Input: part model. Units: mm. Frame: model coordinates. Face numbers are marked on the shaded views. A direction names the side the tool comes from. Round coordinates to 2 decimals unless told otherwise and drop trailing zeros. Order: outer loops, then holes, each group sorted by start corner. A loop starts at its lowest first (then second) coordinate and runs counter-clockwise, first axis right, second up.
Item 1: Cut plane D-D on z = 9.25. Output: boundary loops of the cut face in (x, y).
Item 2: Cut plane B-B on y = 72.5. Output: boundary loops of the cut face in (x, z).
Item 3: Reachability of the marked faces 4, 5 and 6 from +Z, -Z, +X, -X, +Y, -Y: full face, straight path, thin tool, end or side. Return the list, or none.
Item 4: First-contact query: pin 1 (4 mm diameter, centred on x = -3.5, z = 12, fed in from -Y); pin 2 (2 mm diameter, centred on y = 78.5, z = 11.5, fed in from -X); pin 3 (1 mm diameter, centred on x = 5, z = 13, fed in from +Y). Flat tips, straight axial feed; report the tip coordinate or a pass-through.
Item 5: Cut plane A-A on x = -1.5. Output: boundary loops of the cut face in (y, z), then the cut area to 3 significant figures.
Item 6: Mould query, pull axis X, two halves, no side actions, for the marked faces 1, 2 and 3. Classes: released by +X, released by -X, zero draft, split by the parting line, or undercut.
Item 7: Line query: L1, parallel to Z at x = 0.5, y = 63; L2, parallel to X at y = 76, z = 14; L3, parallel to Z at x = -6, y = 67. Output: solid intervals per line, ascending.
Item 8: Cut plane C-C on x = -13. Output: boundary loops of the cut face in (y, z), then the cut area to 3 significant figures.
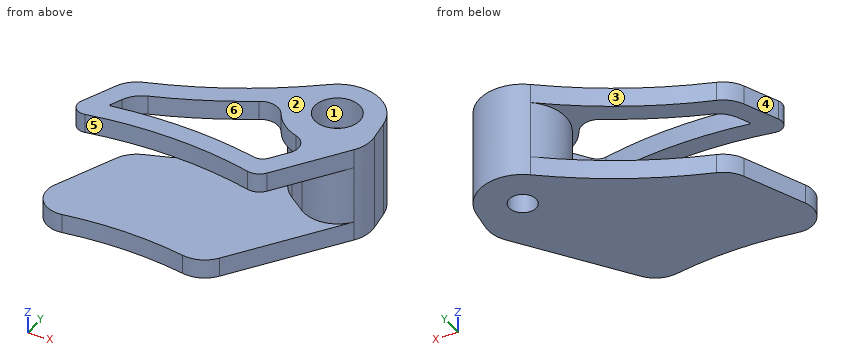
```python
from build123d import *

# Parameters (mm, degrees)
BOSS_EXTRUDE1_DEPTH     = 15
SKETCH16_R              = 2.1
CUT_EXTRUDE2_DEPTH      = 89.504764277
SKETCH17_R              = 3.5
CUT_EXTRUDE3_DEPTH      = 5
CUT_EXTRUDE1_DEPTH      = 5
CUT_EXTRUDE1_DEPTH_BACK = 4
CUT_EXTRUDE5_DEPTH      = 3
CUT_EXTRUDE4_DEPTH      = 3


with BuildPart() as part:
    # Sketch14 → Boss-Extrude1 (new body)
    with BuildSketch(Plane.XY):
        with BuildLine():
            Line((-16.161413536, 57.977264022), (-12.181084948, 67.464973009))
            ThreePointArc((-12.181084948, 67.464973009), (-11.065698538, 69.072353645), (-9.393028071, 70.087209723))
            ThreePointArc((-9.393028071, 70.087209723), (2.046505069, 75.260844547), (12.392283809, 82.373810035))
            ThreePointArc((12.392283809, 82.373810035), (19.046410902, 83.46789097), (23.273577081, 78.213798608))
            Line((23.273577081, 78.213798608), (23.760338244, 74.979563376))
            ThreePointArc((23.760338244, 74.979563376), (23.681286202, 72.988596756), (22.8727833, 71.167465139))
            Line((22.8727833, 71.167465139), (11.475608136, 54.751856173))
            ThreePointArc((11.475608136, 54.751856173), (9.468702378, 53.12015601), (6.90080904, 52.810252891))
            ThreePointArc((6.90080904, 52.810252891), (-2.49021647, 53.523672844), (-11.865953559, 52.631550555))
            ThreePointArc((-11.865953559, 52.631550555), (-15.60520233, 54.025568594), (-16.161413536, 57.977264022))
        make_face()
    extrude(amount=BOSS_EXTRUDE1_DEPTH)

    # Sketch16 → Cut-Extrude2 (cut, through all)
    with BuildSketch(Plane.XY.offset(15)):
        with Locations((16.657019892, 77.21798883)):
            Circle(SKETCH16_R)
    extrude(amount=-CUT_EXTRUDE2_DEPTH, mode=Mode.SUBTRACT)

    # Sketch17 → Cut-Extrude3 (cut)
    with BuildSketch(Plane.XY.offset(15)):
        with Locations((16.657019892, 77.21798883)):
            Circle(SKETCH17_R)
    extrude(amount=-CUT_EXTRUDE3_DEPTH, mode=Mode.SUBTRACT)

    # Sketch15 → Cut-Extrude1 (cut, two sides: drawn at the far end of the back side and taken through both)
    with BuildSketch(Plane.XY.offset(7).offset(-CUT_EXTRUDE1_DEPTH_BACK)):
        with BuildLine():
            Line((13.708420325, 83.2243377), (11.92660987, 87.484761825))
            Line((11.92660987, 87.484761825), (-22.331697338, 87.484761825))
            Line((-22.331697338, 87.484761825), (-22.331697338, 56.566228638))
            Line((-22.331697338, 56.566228638), (-22.331697338, 46.478853626))
            Line((-22.331697338, 46.478853626), (13.179214544, 46.478853626))
            Line((13.179214544, 46.478853626), (31.832474143, 71.167465139))
            Line((31.832474143, 71.167465139), (22.8727833, 71.167465139))
            ThreePointArc((22.8727833, 71.167465139), (19.43169391, 68.968964182), (15.448675977, 69.869003519))
            Line((15.448675977, 69.869003519), (12.782241645, 71.763031479))
            ThreePointArc((12.782241645, 71.763031479), (9.987686622, 77.756932137), (13.708420325, 83.2243377))
        make_face()
    extrude(amount=CUT_EXTRUDE1_DEPTH + CUT_EXTRUDE1_DEPTH_BACK, mode=Mode.SUBTRACT)

    # Sketch19 → Cut-Extrude5 (cut)
    with BuildSketch(Plane.XY.offset(15)):
        with BuildLine():
            Line((-14.431982215, 62.099622447), (-17.748305782, 61.423635141))
            Line((-17.748305782, 61.423635141), (-17.748305782, 50.845501907))
            Line((-17.748305782, 50.845501907), (18.748185883, 50.845501907))
            Line((18.748185883, 50.845501907), (18.748185883, 60.53099213))
            Line((18.748185883, 60.53099213), (15.487998108, 60.53099213))
            ThreePointArc((15.487998108, 60.53099213), (14.424069998, 59.689920639), (13.072075611, 59.582890491))
            ThreePointArc((13.072075611, 59.582890491), (0.311109574, 60.999206641), (-12.463639277, 59.713128338))
            ThreePointArc((-12.463639277, 59.713128338), (-14.168682333, 60.311811806), (-14.431982215, 62.099622447))
        make_face()
    extrude(amount=-CUT_EXTRUDE5_DEPTH, mode=Mode.SUBTRACT)

    # Sketch18 → Cut-Extrude4 (cut)
    with BuildSketch(Plane.XY.offset(15)):
        with BuildLine():
            Line((-9.882439649, 65.189392999), (-10.64394248, 63.374237016))
            ThreePointArc((-10.64394248, 63.374237016), (-10.620440593, 63.202263891), (-10.458545604, 63.139677097))
            ThreePointArc((-10.458545604, 63.139677097), (0.83913118, 63.994498661), (12.110509679, 62.84373919))
            ThreePointArc((12.110509679, 62.84373919), (13.150600921, 62.946203076), (13.96631504, 63.599578248))
            Line((13.96631504, 63.599578248), (15.793536168, 66.231366135))
            ThreePointArc((15.793536168, 66.231366135), (16.091647066, 68.426370752), (14.489067204, 69.955636315))
            ThreePointArc((14.489067204, 69.955636315), (12.025965625, 71.21839557), (10.180541593, 73.281364419))
            ThreePointArc((10.180541593, 73.281364419), (8.387287086, 74.587638576), (6.197252886, 74.232865263))
            ThreePointArc((6.197252886, 74.232865263), (-0.388803899, 70.594783201), (-7.311073103, 67.646228619))
            ThreePointArc((-7.311073103, 67.646228619), (-8.85277752, 66.685766956), (-9.882439649, 65.189392999))
        make_face()
    extrude(amount=-CUT_EXTRUDE4_DEPTH, mode=Mode.SUBTRACT)


solid = part.part
```
From the geometry:
1. outline: (12.78, 71.76) - (15.45, 69.87) arc R5.3 ccw to (23.76, 74.98) - (23.27, 78.21) arc R6.69 ccw (long way) to start; hole circle Ø4.2 at (16.66, 77.22)
2. outline: (-3.38, 0) - (23.54, 0) - (23.54, 15) - (10.73, 15) - (10.73, 12) - (11.91, 12) - (11.91, 3) - (-3.38, 3) - close; (-3.38, 12) - (3.26, 12) - (3.26, 15) - (-3.38, 15) - close
3. face 4: +Z, -Z, -X, +Y
3. face 5: +Z, -Y
3. face 6: +Z
4. pin 1: stops at y = 60.75
4. pin 2: stops at x = 5.95
4. pin 3: stops at y = 77.34
5. outline: (53.52, 0) - (73.39, 0) - (73.39, 3) - (53.52, 3) - close; (60.98, 12) - (63.98, 12) - (63.98, 15) - (60.98, 15) - close; (70.06, 12) - (73.39, 12) - (73.39, 15) - (70.06, 15) - close
5. area: 78.6 mm2
6. face 1: undercut
6. face 2: zero draft
6. face 3: released by -X
7. L1: z = 0 to 3, 12 to 15
7. L2: x = 3.33 to 13.38, 19.94 to 23.61
7. L3: z = 0 to 3
8. outline: (52.59, 0) - (65.51, 0) - (65.51, 3) - (52.59, 3) - close; (59.69, 12) - (65.51, 12) - (65.51, 15) - (59.69, 15) - close
8. area: 56.2 mm2
